Autodesk Inventor part; units mm, degrees
ref_plane "YZ Plane" through (0, 0, 0) normal (1, 0, 0) x (0, 1, 0)
ref_plane "XZ Plane" through (0, 0, 0) normal (0, 1, 0) x (-1, 0, 0)
ref_plane "XY Plane" through (0, 0, 0) normal (0, 0, 1) x (1, 0, 0)
sketch "Sketch1" plane through (0, 0, 0) normal (0, 0, 1) x (1, 0, 0)
  line L0 (0, 0) -> (0, 12.7)
  line L1 (0, 12.7) -> (-31.75, 12.7)
  line L2 (-31.75, 12.7) -> (-31.75, 7.9375)
  line L3 (-31.75, 7.9375) -> (-4.7625, 7.9375)
  line L4 (-4.7625, 7.9375) -> (-4.7625, 0)
  line L5 (0, 0) -> (0, -12.7)
  line L6 (0, -12.7) -> (-31.75, -12.7)
  line L7 (-31.75, -12.7) -> (-31.75, -7.9375)
  line L8 (-31.75, -7.9375) -> (-4.7625, -7.9375)
  line L9 (-4.7625, -7.9375) -> (-4.7625, 0)
  dimension "width" = 25.4
  dimension "thickness" = 4.7625
  dimension "d2" = 4.7625
  dimension "height" = 31.75
extrude "Extrusion1" add sketch "Sketch1" along normal mid plane 406.4
equation "\"d2\" = thickness"
properties part number "1 x 16 x 3_16" material "Aluminum 6061"
Source: CAD feature listing. Evaluate the final solid. Frame: model axes, mm. A direction names the side the tool comes from. Round coordinates to 2 decimals unless told otherwise and drop trailing zeros. Loops run counter-clockwise (first coordinate to the right, second up) from the corner with the lowest first, then second, coordinate; pieces in that order, holes last. Notation, with made-up numbers: M -33,16 L 10,16 A16 ccw 10,46 Z; hole C -22.75,12.25 d10. An arc over 180 degrees is marked long. Use a Markdown table: item, result. Add a question column.
1. Section query B-B on z = -167. Return the cut outline in (x, y), then the cut area to 3 significant figures.
2. Section query C-C on y = 3.75. Return the cut outline in (x, z).
3. Section query A-A on x = -24.5. Return the cut outline in (y, z).
4. Reachability of faces 1 (the flat face through (-18, -7.938, -3)), 2 (the flat face through (-16, -12.7, -3)) from +Z, -Z, +X, -X, +Y, -Y: full face, straight path, thin tool, end or side. Return the list, or none.
5. Mould query, pull axis Y, two halves, no side actions, for faces 3 (the flat face through (0, 0, -3)), 4 (the flat face through (-18, 7.938, -3)), 5 (the flat face through (-16, 12.7, -3)). Classes: pulls with the +Y half, pulls with the -Y half, needs draft (parallel to the pull), parting line crosses it, or undercut.
6. Line query: line 1 (Y direction, x = -21, z = 106); line 2 (X direction, y = 5.5, z = 137). Output: solid intervals per line, ascending.
7. Contact query for flat-ended pins moving along their axis: P1, Ø3, axis at y = -2.5, z = -34, coming from the +X side; P2, Ø5, axis at y = 0, z = 72, coming from the -X side. Output: stop coordinate, or through.
Reported:
| question | item | result |
|---|---|---|
| 1 | outline | M -31.75,-12.7 L 0,-12.7 L 0,12.7 L -31.75,12.7 L -31.75,7.94 L -4.76,7.94 L -4.76,-7.94 L -31.75,-7.94 Z |
| 1 | area | 378 mm² |
| 2 | outline | M -4.76,-203.2 L 0,-203.2 L 0,203.2 L -4.76,203.2 Z |
| 3 | outline | M -12.7,-203.2 L -7.94,-203.2 L -7.94,203.2 L -12.7,203.2 Z; M 7.94,-203.2 L 12.7,-203.2 L 12.7,203.2 L 7.94,203.2 Z |
| 4 | face 1 | +Z, -Z, -X |
| 4 | face 2 | +Z, -Z, +X, -X, -Y |
| 5 | face 3 | needs draft |
| 5 | face 4 | undercut |
| 5 | face 5 | pulls with the +Y half |
| 6 | line 1 | y = -12.7 to -7.94, 7.94 to 12.7 |
| 6 | line 2 | x = -4.76 to 0 |
| 7 | P1 | stops at x = 0 |
| 7 | P2 | stops at x = -4.76 |
